The listing builds one solid part. Answer for the finished solid, in the listing's coordinates (mm). A direction names the side the tool comes from. Give positions to 0.01 mm unless a question says otherwise; leave off trailing zeros. Write each loop counter-clockwise with the first axis right and the second up, starting at its lowest first coordinate (ties: lowest second). Pieces come first, ordered by that corner, then holes. Notation, with made-up numbers: M 22,40.25 L 51,40.25 A20 ccw 51,76.25 Z; hole C 40.25,12 d5. An arc over 180 degrees is marked long. Return JSON: item names as keys, results as strings.
Autodesk Inventor part; units mm, degrees
ref_plane "YZ Plane" through (0, 0, 0) normal (1, 0, 0) x (0, 1, 0)
ref_plane "XZ Plane" through (0, 0, 0) normal (0, 1, 0) x (-1, 0, 0)
ref_plane "XY Plane" through (0, 0, 0) normal (0, 0, 1) x (1, 0, 0)
sketch "スケッチ1" plane through (0, 0, 0) normal (0, 0, 1) x (1, 0, 0)
  line L0 (-12.5, 12.5) -> (12.5, 12.5)
  line L1 (12.5, 12.5) -> (12.5, -12.5)
  line L2 (12.5, -12.5) -> (-12.5, -12.5)
  line L3 (-12.5, -12.5) -> (-12.5, 12.5)
  line L4 (-12.5, 12.5) -> (12.5, -12.5) construction
  line L5 (12.5, 12.5) -> (-12.5, -12.5) construction
  point P0 (0, 0)
  dimension "d0" = 25
  dimension "d1" = 25
extrude "押し出し1" add sketch "スケッチ1" along normal mid plane 50
shell "シェル1" thickness 2.3 removed faces 2 at (-4.1667, -4.1667, 25) at (-4.1667, -4.1667, -25)
sketch "スケッチ2" plane through (12.5, -12.5, 25) normal (1, 0, 0) x (0, 0, -1)
  line L0 (0, 22.7) -> (20, 22.7)
  line L1 (20, 22.7) -> (20, 2.3)
  line L2 (20, 2.3) -> (0, 2.3)
  line L3 (0, 2.3) -> (0, 22.7)
  line L4 (0, 22.7) -> (20, 2.3) construction
  line L5 (20, 22.7) -> (0, 2.3) construction
  line L6 (0, 0) -> (0, 25)
  point P0 (25, 12.5)
  point P1 (10, 12.5)
  dimension "d5" = 20
extrude "押し出し2" cut sketch "スケッチ2" against normal through all
sketch "スケッチ3" plane through (-12.5, 12.5, 25) normal (0, 1, 0) x (1, 0, 0)
  circle A0 centre (12.5, 10) radius 4
  line L0 (25, 0) -> (0, 0)
  line L1 (0, 50) -> (0, 0)
  point P0 (12.5, 25)
  dimension "d8" = 8
  dimension "d9" = 10
  dimension "d10" = 12.5
extrude "押し出し3" cut sketch "スケッチ3" against normal through all
fillet "フィレット1" radius 7 8 edges at (12.5, -11.35, 25) (-12.5, -11.35, 25) (-12.5, 11.35, 25) (12.5, 11.35, 25) (11.35, 10.2, 5) (-11.35, 10.2, 5) (-11.35, -10.2, 5) (11.35, -10.2, 5)
equation "\"d1\" = d0"
properties part number "body-braket"
Item 1: Find the intervals of material crossed by line 1 (Y direction, x = 7.5, z = -17); line 2 (X direction, y = -11.05, z = 15), in increasing order.
Geometry results:
{"line 1": "y = -12.5 to -10.2, 10.2 to 12.5", "line 2": "x = -12.5 to -4, 4 to 12.5"}
Item 2: A cutting plane is placed at B-B, the plane x = 0. Write down the section's boundary in (y, z).
Geometry results:
{"outline": "M -12.5,-25 L -10.2,-25 L -10.2,11 L -12.5,11 Z; M -12.5,19 L -10.2,19 L -10.2,25 L -12.5,25 Z; M 10.2,-25 L 12.5,-25 L 12.5,11 L 10.2,11 Z; M 10.2,19 L 12.5,19 L 12.5,25 L 10.2,25 Z"}
Item 3: A cutting plane is placed at D-D, the plane z = 3. Write down the section's boundary in (x, y).
Geometry results:
{"outline": "M -12.5,-12.5 L 12.5,-12.5 L 12.5,12.5 L -12.5,12.5 Z; hole M -10.2,-10.2 L 10.2,-10.2 L 10.2,10.2 L -10.2,10.2 Z"}
Item 4: Which of the six approach directions +Z, -Z, +X, -X, +Y, -Y give full straight-line access (tool end or side, diameter ignored) to faces 4 (the cylindrical face through (-0.521, 11.366, 11.034)), 5 (the flat face through (-11, 0, 5)), 6 (the flat face through (-10.2, 0, -11))?
Geometry results:
{"face 4": "+Y, -Y", "face 5": "+Z, +X, -X", "face 6": "+Z, -Z"}
Item 5: A cutting plane is placed at C-C, the plane y = 0.75. Write down the section's boundary in (x, z).
Geometry results:
{"outline": "M -12.5,-25 L -10.2,-25 L -10.2,5 L -12.5,5 Z; M 10.2,-25 L 12.5,-25 L 12.5,5 L 10.2,5 Z"}
Item 6: A cutting plane is placed at A-A, the plane z = 15. Write down the section's boundary in (x, y), plus the area to 3 significant figures.
Geometry results:
{"outline": "M -12.5,-12.5 L -4,-12.5 L -4,-10.2 L -12.5,-10.2 Z; M -12.5,10.2 L -4,10.2 L -4,12.5 L -12.5,12.5 Z; M 4,-12.5 L 12.5,-12.5 L 12.5,-10.2 L 4,-10.2 Z; M 4,10.2 L 12.5,10.2 L 12.5,12.5 L 4,12.5 Z", "area": "78.2 mm2"}
Item 7: Determine the mould class of faces 1 (the cylindrical face through (-11.4, -8.1, 7)), 2 (the flat face through (0, 12.5, 0)), 3 (the cylindrical face through (-10.5, -11.3, 22.9)) for opening direction Y: +Y half, -Y half, draft (parallel to the pull), parting line (faces both ways), or undercut.
Geometry results:
{"face 1": "undercut", "face 2": "+Y half", "face 3": "draft"}
Item 8: Given pin 1 Ø6 at (x, y) = (-5.5, -6.5) entering from +Z; pin 2 Ø1.8 at (x, y) = (-12, 1) entering from +Z, each flat-ended and moving along its own axis, determine where each tip first touches the part or whether it passes through.
Geometry results:
{"pin 1": "passes through", "pin 2": "stops at z = 5"}
